Geometry: final body of the model. Coordinates: model frame, mm. Coordinates: 2 decimals unless noted, no trailing zeros. Write each loop counter-clockwise with the first axis right and the second up, starting at its lowest first coordinate (ties: lowest second). Pieces come first, ordered by that corner, then holes. Notation, with made-up numbers: M 19,-3 L 58,-3 A18 cw 58,24 Z; hole C 10.25,-4.75 d11. An arc over 180 degrees is marked long. Write item = value, one per line. Start each with the question number.
Item 1: Section B-B on y = 2.3. Give the number of separate pieces and of enclosed holes in the cut face, plus the area to 3 significant figures.
Item 2: Ray query, L1, parallel to X at y = 1.85, z = -33.5; L2, parallel to Z at x = 129, y = 3.3; L3, parallel to X at y = 4.5, z = -170. Return the intervals inside material, ascending. Write a range as [from, to].
Item 3: Section A-A on z = -161. Output: boundary loops of the cut face in (x, y), plus the area to 3 significant figures.
Autodesk Inventor part; units mm, degrees
ref_plane "YZ Plane" through (0, 0, 0) normal (1, 0, 0) x (0, 1, 0)
ref_plane "XZ Plane" through (0, 0, 0) normal (0, 1, 0) x (-1, 0, 0)
ref_plane "XY Plane" through (0, 0, 0) normal (0, 0, 1) x (1, 0, 0)
sketch "Sketch1" plane through (0, 0, 0) normal (0, 1, 0) x (-1, 0, 0)
  line L0 (0, 0) -> (-280, 0)
  line L1 (-280, 0) -> (-280, -270)
  line L2 (-280, -270) -> (0, -270)
  line L3 (0, -270) -> (0, 0)
  line L4 (0, -135) -> (-280, -135) construction
  line L5 (-140, 0) -> (-140, -270) construction
  line L6 (-70, 0) -> (-70, -270) construction
  line L7 (-210, 0) -> (-210, -270) construction
  line L8 (-30, -240) -> (-30, -210) construction
  line L9 (-30, -240) -> (-30, -210) construction
  line L10 (-27.75, -240) -> (-27.75, -210)
  line L11 (-32.25, -210) -> (-32.25, -240)
  arc A0 (-32.25, -240) -> (-27.75, -240) centre (-30, -240) ccw
  arc A1 (-27.75, -210) -> (-32.25, -210) centre (-30, -210) ccw
  line L12 (-110, -240) -> (-110, -210) construction
  line L13 (-110, -240) -> (-110, -210) construction
  line L14 (-112.25, -240) -> (-112.25, -210)
  line L15 (-107.75, -210) -> (-107.75, -240)
  arc A2 (-112.25, -240) -> (-107.75, -240) centre (-110, -240) ccw
  arc A3 (-107.75, -210) -> (-112.25, -210) centre (-110, -210) ccw
  line L16 (-160, -260) -> (-120, -260)
  line L17 (-120, -260) -> (-120, -254.7)
  line L18 (-120, -254.7) -> (-160, -254.7)
  line L19 (-160, -254.7) -> (-160, -260)
  line L20 (-250, -240) -> (-250, -210) construction
  line L21 (-250, -240) -> (-250, -210) construction
  line L22 (-252.25, -240) -> (-252.25, -210)
  line L23 (-247.75, -210) -> (-247.75, -240)
  arc A4 (-252.25, -240) -> (-247.75, -240) centre (-250, -240) ccw
  arc A5 (-247.75, -210) -> (-252.25, -210) centre (-250, -210) ccw
  line L24 (-172.25, -210) -> (-172.25, -240)
  line L25 (-170, -240) -> (-170, -210) construction
  line L26 (-167.75, -240) -> (-167.75, -210)
  arc A6 (-172.25, -240) -> (-167.75, -240) centre (-170, -240) ccw
  line L27 (-170, -240) -> (-170, -210) construction
  arc A7 (-167.75, -210) -> (-172.25, -210) centre (-170, -210) ccw
  line L28 (-140, -270) -> (-140, 0) construction
  line L29 (-30, -30) -> (-30, -60) construction
  line L30 (-30, -30) -> (-30, -60) construction
  line L31 (-27.75, -30) -> (-27.75, -60)
  line L32 (-32.25, -60) -> (-32.25, -30)
  arc A8 (-27.75, -30) -> (-32.25, -30) centre (-30, -30) ccw
  arc A9 (-32.25, -60) -> (-27.75, -60) centre (-30, -60) ccw
  line L33 (-107.75, -60) -> (-107.75, -30)
  line L34 (-110, -30) -> (-110, -60) construction
  line L35 (-112.25, -30) -> (-112.25, -60)
  arc A10 (-107.75, -30) -> (-112.25, -30) centre (-110, -30) ccw
  line L36 (-110, -30) -> (-110, -60) construction
  arc A11 (-112.25, -60) -> (-107.75, -60) centre (-110, -60) ccw
  line L37 (-160, -10) -> (-120, -10)
  line L38 (-120, -10) -> (-120, -15.3)
  line L39 (-120, -15.3) -> (-160, -15.3)
  line L40 (-160, -15.3) -> (-160, -10)
  arc A12 (-247.75, -30) -> (-252.25, -30) centre (-250, -30) ccw
  line L41 (-247.75, -60) -> (-247.75, -30)
  line L42 (-250, -30) -> (-250, -60) construction
  line L43 (-250, -30) -> (-250, -60) construction
  arc A13 (-252.25, -60) -> (-247.75, -60) centre (-250, -60) ccw
  line L44 (-252.25, -30) -> (-252.25, -60)
  line L45 (-172.25, -60) -> (-172.25, -30)
  line L46 (-170, -30) -> (-170, -60) construction
  line L47 (-170, -30) -> (-170, -60) construction
  arc A14 (-172.25, -60) -> (-167.75, -60) centre (-170, -60) ccw
  line L48 (-167.75, -30) -> (-167.75, -60)
  arc A15 (-167.75, -30) -> (-172.25, -30) centre (-170, -30) ccw
  line L49 (-270, -95) -> (-270, -145)
  line L50 (-270, -145) -> (-270, -180)
  line L51 (-270, -180) -> (-264.7, -180)
  line L52 (-264.7, -180) -> (-264.7, -80)
  line L53 (-264.7, -80) -> (-270, -80)
  line L54 (-270, -80) -> (-270, -95)
  line L55 (0, -90) -> (-5.3, -90)
  line L56 (-5.3, -90) -> (-5.3, -190)
  line L57 (-5.3, -190) -> (0, -190)
  line L58 (0, -190) -> (0, -90)
  point P0 (-30, -225)
  point P1 (-110, -225)
  point P2 (-250, -225)
  point P3 (-170, -225)
  point P4 (-30, -45)
  point P5 (-110, -45)
  point P6 (-250, -45)
  point P7 (-170, -45)
  point P8 (0, -190)
  dimension "d0" = 280
  dimension "d1" = 270
  dimension "d2" = 30
  dimension "d3" = 40
  dimension "d4" = 30
  dimension "d6" = 2.25
  dimension "d9" = 40
  dimension "d13" = 10
  dimension "d14" = 5.3
  dimension "d16" = 20
  dimension "d20" = 10
  dimension "d21" = 5.3
  dimension "d22" = 5.3
extrude "Extrusion1" add sketch "Sketch1" along normal blind 5 contours L3 L55 L56 L57 L2 L1 L0
properties part number "base_2"
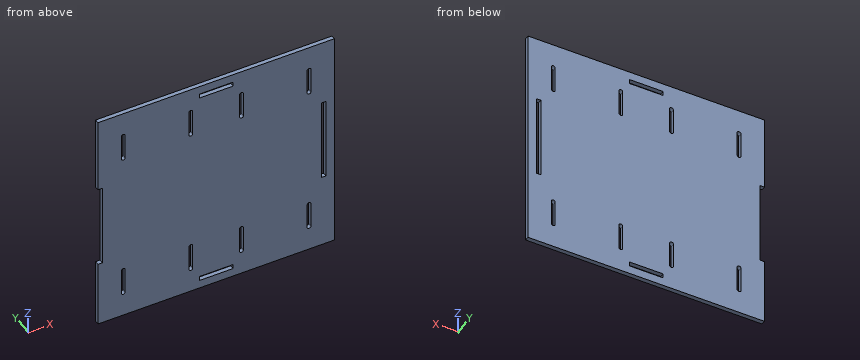
Responses:
q1.separate_pieces = 1
q1.enclosed_holes = 11
q1.area = 72,900 mm²
q2.L1 = [0, 27.75], [32.25, 107.75], [112.25, 167.75], [172.25, 247.75], [252.25, 280]
q2.L2 = [-270, -260], [-254.7, -15.3], [-10, 0]
q2.L3 = [5.3, 264.7], [270, 280]
q3.outline = M 5.3,0 L 264.7,0 L 264.7,5 L 5.3,5 Z; M 270,0 L 280,0 L 280,5 L 270,5 Z
q3.area = 1,350 mm²
